Part model, mm, in its own coordinate system. A direction names the side the tool comes from. Coordinates: 2 decimals unless noted, no trailing zeros. Order: outer loops, then holes, each group sorted by start corner. A loop starts at its lowest first (then second) coordinate and runs counter-clockwise, first axis right, second up.
1) Pin check, flat tips, straight feed: pin 1 Ø10 at (x, z) = (-5, 6.5) entering from +Y; pin 2 Ø5 at (y, z) = (11, 20) entering from +X; pin 3 Ø1 at (x, y) = (73.5, -0.5) entering from -Z; pin 4 Ø12 at (x, y) = (-28.5, -50.5) entering from -Z. Stop position of each tip, or through.
2) Wall check: L1, parallel to X at y = -29.5, z = 7.5; L2, parallel to Y at x = -16, z = 11.25; L3, parallel to Z at x = 90.5, y = -2. Give the ranges that are in metal, low to high.
3) Cut at C-C (y = 9). List the corners of the cut face in (x, z), and give its area (3 significant figures).
4) Cut at A-A (x = 86). List the corners of the cut face in (y, z).
5) Tool access for faces 1 (the flat face through (54, 26.134, 22)), 2 (the flat face through (52, -22.301, 22)), 3 (the flat face through (119, 2, 12.7)), 4 (the cylindrical face through (109, 4, 7)), 5 (the flat face through (-80.033, 1, 6)): list every direction of +Z, -Z, +X, -X, +Y, -Y with a clear straight run to the whole face (end or side of a thin tool).
6) Cut at D-D (y = 52.5). List the corners of the cut face in (x, z).
7) Cut at B-B (z = 2.5). List the corners of the cut face in (x, y), and give its area (3 significant figures).
8) Mould opens along Y. For faces 6 (the flat face through (52, 2, 25.4)), 7 (the flat face through (-16.73, -41.07, 6.26)), 8 (the flat face through (-9.97, 57.6, 6.26)) say: +Y half, -Y half, draft (parallel to the pull), parting line (faces both ways), or undercut.
```python
from build123d import *

# Parameters (mm, degrees)
F3_DEPTH = 12.7
F5_DEPTH = 12.7
F6_DEPTH = 5


# Not quite as in the source:
# - a feature names something its author has since deleted; it is built from what else it names


with BuildPart() as f3:
    # F2 (on Top) → F3 (new body)
    with BuildSketch(Plane.XY):
        with BuildLine():
            Line((-3.986357704, 43.8342139564), (-16.1254491208, 71.7667039931))
            Line((-16.1254491208, 71.7667039931), (-92.733014825, 71.7667039931))
            Line((-92.733014825, 71.7667039931), (-92.733014825, -67.9332960069))
            Line((-92.733014825, -67.9332960069), (-16.1254491208, -67.9332960069))
            Line((-16.1254491208, -67.9332960069), (-3.986357704, -40.0008059702))
            ThreePointArc((-3.986357704, -40.0008059702), (121.738009035, 1.9167039931), (-3.986357704, 43.8342139564))
        make_face()
        with BuildLine():
            Line((-80.033014825, -55.2332960069), (-80.033014825, 59.0667039931))
            Line((-80.033014825, 59.0667039931), (-22.883014825, 59.0667039931))
            Line((-22.883014825, 59.0667039931), (-10.7439288273, 31.1342139564))
            Line((-10.7439288273, 31.1342139564), (2.7712134193, 31.1342139564))
            ThreePointArc((2.7712134193, 31.1342139564), (109.038009035, 1.9167039931), (2.7712134193, -27.3008059702))
            Line((2.7712134193, -27.3008059702), (-10.7439288273, -27.3008059702))
            Line((-10.7439288273, -27.3008059702), (-22.883014825, -55.2332960069))
            Line((-22.883014825, -55.2332960069), (-80.033014825, -55.2332960069))
        make_face(mode=Mode.SUBTRACT)
    extrude(amount=F3_DEPTH)

    # F4 (on face) → F5 (join)
    with BuildSketch(Plane.XY.offset(12.7)):
        with BuildLine():
            Line((103.6531972523, 26.1342139564), (-10.7439288273, 26.1342139564))
            Line((-10.7439288273, 26.1342139564), (-10.7439288273, -22.3008059702))
            Line((-10.7439288273, -22.3008059702), (103.6531972523, -22.3008059702))
            ThreePointArc((103.6531972523, -22.3008059702), (109.038009035, 1.9167039931), (103.6531972523, 26.1342139564))
        make_face()
        with BuildLine():
            Line((117.405447257, 26.1342139564), (103.6531972523, 26.1342139564))
            ThreePointArc((103.6531972523, 26.1342139564), (109.038009035, 1.9167039931), (103.6531972523, -22.3008059702))
            Line((103.6531972523, -22.3008059702), (117.405447257, -22.3008059702))
            Line((117.405447257, -22.3008059702), (117.405447257, 26.1342139564))
        make_face()
    extrude(amount=F5_DEPTH)

    # F6 (cut): a face of the model
    f6_faces = [f3.faces().sort_by_distance(p)[0] for p in [
        (48.2779564243, 1.9167039931, 12.7),
    ]]
    extrude(f6_faces, amount=-F6_DEPTH, mode=Mode.SUBTRACT)


solid = f3.part
```
Geometry check:
1. pin 1: stops at y = 57.67
1. pin 2: stops at x = 117.41
1. pin 3: stops at z = 17.7
1. pin 4: stops at z = 0
2. L1: x = -92.73 to -80.03, -11.7 to 4.15, 99.63 to 114.27
2. L2: y = -67.64 to -39.4, 43.23 to 71.48
2. L3: z = 17.7 to 25.4
3. outline: (-92.73, 0) - (-80.03, 0) - (-80.03, 12.7) - (-92.73, 12.7) - close; (-10.74, 17.7) - (108.6, 17.7) - (108.6, 0) - (121.38, 0) - (121.38, 12.7) - (117.41, 12.7) - (117.41, 25.4) - (-10.74, 25.4) - close
3. area: 1,350 mm2
4. outline: (-59.04, 0) - (-43.94, 0) - (-43.94, 12.7) - (-59.04, 12.7) - close; (-22.3, 17.7) - (26.13, 17.7) - (26.13, 25.4) - (-22.3, 25.4) - close; (47.77, 0) - (62.87, 0) - (62.87, 12.7) - (47.77, 12.7) - close
5. face 1: +Z, +X, -X, +Y
5. face 2: +Z, +X, -X, -Y
5. face 3: +Z, +X, +Y, -Y
5. face 4: -Z
5. face 5: +Z, -Z
6. outline: (-92.73, 0) - (-80.03, 0) - (-80.03, 12.7) - (-92.73, 12.7) - close; (-20.03, 0) - (-7.75, 0) - (-7.75, 12.7) - (-20.03, 12.7) - close; (3.72, 0) - (25.29, 0) - (25.29, 12.7) - (3.72, 12.7) - close; (78.49, 0) - (100.06, 0) - (100.06, 12.7) - (78.49, 12.7) - close
7. outline: (-92.73, -67.93) - (-16.13, -67.93) - (-3.99, -40) arc R69.85 ccw (long way) to (-3.99, 43.83) - (-16.13, 71.77) - (-92.73, 71.77) - close; hole (-80.03, -55.23) - (-22.88, -55.23) - (-10.74, -27.3) - (2.77, -27.3) arc R57.15 ccw (long way) to (2.77, 31.13) - (-10.74, 31.13) - (-22.88, 59.07) - (-80.03, 59.07) - close
7. area: 8,270 mm2
8. face 6: draft
8. face 7: undercut
8. face 8: +Y half
